The listing builds one solid part. Answer for the finished solid, in the listing's coordinates (mm). A direction names the side the tool comes from. Coordinates: 2 decimals unless noted, no trailing zeros. Order: outer loops, then holes, each group sorted by start corner. A loop starts at its lowest first (then second) coordinate and runs counter-clockwise, first axis right, second up. Notation, with made-up numbers: (64.5, 86.25) -> (73.5, 86.25) arc R12 ccw to (73.5, 105.25) -> close; hole circle Ø4 at (-14, 38.25). An arc over 180 degrees is marked (long way). Write item = value, one per line.
from build123d import *

# Parameters (mm, degrees)
SZKIC1_R                    = 3
DODANIE_WYCI_GNI_CIE1_DEPTH = 20.5
WYTNIJ_WYCI_GNI_CIE1_START  = -1.8
SZKIC2_R                    = 3
SZKIC2_R_2                  = 2.85
WYTNIJ_WYCI_GNI_CIE1_DEPTH  = 0.8
WYTNIJ_WYCI_GNI_CIE2_START  = -19.5
SZKIC2_2_R                  = 3
SZKIC2_2_R_2                = 2.85
WYTNIJ_WYCI_GNI_CIE2_DEPTH  = 0.8
SFAZOWANIE1_SIZE            = 0.5


with BuildPart() as part:
    # Szkic1 → Dodanie-wyciągnięcie1 (new body)
    with BuildSketch(Plane.XY):
        Circle(SZKIC1_R)
    extrude(amount=DODANIE_WYCI_GNI_CIE1_DEPTH)

    # Szkic2 → Wytnij-wyciągnięcie1 (cut)
    with BuildSketch(Plane.XY.offset(20.5).offset(WYTNIJ_WYCI_GNI_CIE1_START)):
        Circle(SZKIC2_R)
        Circle(SZKIC2_R_2, mode=Mode.SUBTRACT)
    extrude(amount=WYTNIJ_WYCI_GNI_CIE1_DEPTH, mode=Mode.SUBTRACT)

    # Szkic2<2> → Wytnij-wyciągnięcie2 (cut)
    with BuildSketch(Plane.XY.offset(20.5).offset(WYTNIJ_WYCI_GNI_CIE2_START)):
        Circle(SZKIC2_2_R)
        Circle(SZKIC2_2_R_2, mode=Mode.SUBTRACT)
    extrude(amount=WYTNIJ_WYCI_GNI_CIE2_DEPTH, mode=Mode.SUBTRACT)

    # Sfazowanie1
    sfazowanie1_edges = [part.edges().sort_by_distance(p)[0] for p in [
        (-3, 0, 0),
        (-3, 0, 20.5),
    ]]
    chamfer(sfazowanie1_edges, length=SFAZOWANIE1_SIZE)


solid = part.part
Q1. The mould has two halves that part along Z. Classify faces 3 (the face through (-3, 0.1, 0.7)), 4 (the face through (0, 0, 20.5)), 5 (the face through (-2.262, -1.734, 19.094)): released by +Z, released by -Z, zero draft, split by the parting line, or undercut.
The answers:
face_3 = zero draft
face_4 = released by +Z
face_5 = undercut
Q2. Section A-A, the plane z = 1.5 is taken. Give the vertices of the cut face in (x, y), plus the area to 3 significant figures.
The answers:
outline = circle Ø5.7 at (0, 0)
area = 25.5 mm2
Q3. Find the intervals of material crossed by line 1 along X through (y, z) = (0.1, 12.75); line 2 along Y through (x, z) = (1.6, 8), in increasing order.
The answers:
line_1 = -3 to 3
line_2 = -2.54 to 2.54
Q4. A tool of negligible diameter and unlimited length cuts with its end or side. For faces 1 (the face through (-3, 0, 10)), 2 (the face through (-2.262, -1.734, 1.394)), from which of +Z, -Z, +X, -X, +Y, -Y can it reach the whole face along a straight path? Write none if from no direction.
The answers:
face_1 = +Z, -Z
face_2 = none
Q5. Each of these flat-tipped pins is pushed along its axis until it touches: pin 1 Ø2 at (x, z) = (-2.5, 14) entering from -Y; pin 2 Ø1.8 at (x, y) = (1, 0.5) entering from -Z; pin 3 Ø1.5 at (x, z) = (1.5, 13.5) entering from -Y. Where does it stop, or does it pass through?
The answers:
pin_1 = -2.6
pin_2 = 0
pin_3 = -2.9
Q6. Section B-B, the plane z = 16.25 is taken. Give the vertices of the cut face in (x, y).
The answers:
outline = circle Ø6 at (0, 0)
